Input: part model. Units: mm. Frame: model coordinates. Face numbers are marked on the shaded views. A direction names the side the tool comes from. Give positions to 0.01 mm unless a question says otherwise; leave off trailing zeros. Order: outer loops, then holes, each group sorted by start corner. A loop starts at its lowest first (then second) coordinate and runs counter-clockwise, first axis right, second up. Notation, with made-up numbers: M -13,5 L -5,5 A20 cw -5,32 Z; hole C 42.5,-12.75 d4. An arc over 180 degrees is marked long. Use a Markdown table: item, result.
from build123d import *

# Parameters (mm, degrees)
F0_W     = 42
F0_H     = 42
F0_R     = 10.5
F1_DEPTH = 4
F2_DEPTH = 57
F3_R     = 5


with BuildPart() as f1:
    # F0 (on Top) → F1 (new body)
    with BuildSketch(Plane.XY):
        with Locations((-0.312906, -0.03483)):
            Rectangle(F0_W, F0_H)
        Circle(F0_R, mode=Mode.SUBTRACT)
        Circle(F0_R)
    extrude(amount=F1_DEPTH)

    # F0 (on Top) → F2 (join)
    with BuildSketch(Plane.XY):
        Circle(F0_R)
    extrude(amount=F2_DEPTH)

    # F3
    f3_edges = [f1.edges().sort_by_distance(p)[0] for p in [
        (-21.312906, -21.03483, 2),
        (-21.312906, 20.96517, 2),
        (20.687094, -21.03483, 2),
        (20.687094, 20.96517, 2),
    ]]
    fillet(f3_edges, radius=F3_R)


solid = f1.part
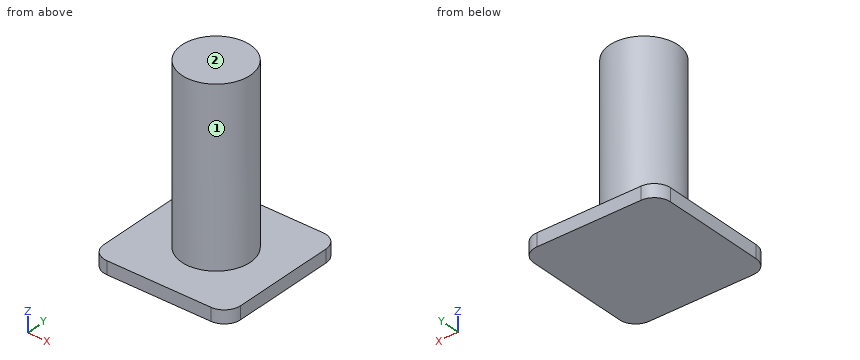
1) Reachability of the marked faces 1 and 2 from +Z, -Z, +X, -X, +Y, -Y: full face, straight path, thin tool, end or side. Return the list, or none.
Response values:
| item | result |
|---|---|
| face 1 | +Z |
| face 2 | +Z, +X, -X, +Y, -Y |
2) Material intervals for line 1 (Z direction, x = 15, y = 9); line 2 (X direction, y = -0.5, z = 39.5); line 3 (X direction, y = -6, z = 45.5), sorted ascending. Write a range as from..to.
Response values:
| item | result |
|---|---|
| line 1 | z = 0..4 |
| line 2 | x = -10.49..10.49 |
| line 3 | x = -8.62..8.62 |
3) Cut plane D-D on y = -12. Return loops of the section in (x, z), and give its area (3 significant figures).
Response values:
| item | result |
|---|---|
| outline | M -21.31,0 L 20.69,0 L 20.69,4 L -21.31,4 Z |
| area | 168 mm² |
4) Cut plane A-A on x = 0. Return loops of the section in (y, z), and give its area (3 significant figures).
Response values:
| item | result |
|---|---|
| outline | M -21.03,0 L 20.97,0 L 20.97,4 L 10.5,4 L 10.5,57 L -10.5,57 L -10.5,4 L -21.03,4 Z |
| area | 1,280 mm² |
5) First-contact query: pin 1 Ø1 at (x, y) = (-7.5, 1.5) entering from -Z; pin 2 Ø2 at (y, z) = (1.5, 26.5) entering from +X; pin 3 Ø12 at (x, z) = (-12.5, 18) entering from +Y; pin 4 Ø12 at (y, z) = (13.5, 40) entering from -X. Flat tips, straight axial feed; report the tip coordinate or a pass-through.
Response values:
| item | result |
|---|---|
| pin 1 | stops at z = 0 |
| pin 2 | stops at x = 10.49 |
| pin 3 | stops at y = 8.25 |
| pin 4 | stops at x = -7.35 |
6) Cut plane B-B on y = 0. Return loops of the section in (x, z), and give its area (3 significant figures).
Response values:
| item | result |
|---|---|
| outline | M -21.31,0 L 20.69,0 L 20.69,4 L 10.5,4 L 10.5,57 L -10.5,57 L -10.5,4 L -21.31,4 Z |
| area | 1,280 mm² |
7) Cut plane C-C on z = 29. Return loops of the section in (x, y), and give its area (3 significant figures).
Response values:
| item | result |
|---|---|
| outline | C 0,0 d21 |
| area | 346 mm² |
